Study the drawing (mm; zero at the part's minimum x, y, z) and answer. A direction names the side the tool comes from. Coordinates: 2 decimals unless noted, no trailing zeros. Loops run counter-clockwise (first coordinate to the right, second up) from the corner with the lowest first, then second, coordinate; pieces in that order, holes last.
Q1. Section C-C (x = 8.5) is taken. Give the vertices of the cut face in (y, z).
Q2. The mould has two halves that part along X. Classify the marked faces 3, 4 and 5: pulls with the +X half, pulls with the -X half, needs draft (parallel to the pull), parting line crosses it, or undercut.
Q3. Which of the six approach directions +Z, -Z, +X, -X, +Y, -Y give full straight-line access (tool end or side, diameter ignored) to the marked faces 1 and 2?
Q4. Flat-ended cylindrical pins translate along their axes: P1, Ø1.5, axis at x = 38, y = 18.5, coming from the +Z side; P2, Ø1.8, axis at x = 4, z = 21, coming from the +Y side; P3, Ø5, axis at x = 18.5, y = 4, coming from the +Z side; P4, Ø10.5, axis at x = 41.5, z = 14.5, coming from the +Y side. Find the tip coordinate at first contact, or state that the pin passes through.
Q5. Section A-A (y = 16) is taken. Give the vertices of the cut face in (x, z), then the cut area to 3 significant figures.
Q6. Section B-B (z = 23.5) is taken. Give the vertices of the cut face in (x, y).
Q7. Straight lines are drawn through the part: line 1 (X direction, y = 8.5, z = 28); line 2 (Y direction, x = 52, z = 4.5); line 3 (Y direction, x = 52, z = 20.5). For each, find the intervals that lie inside material, in ascending order.
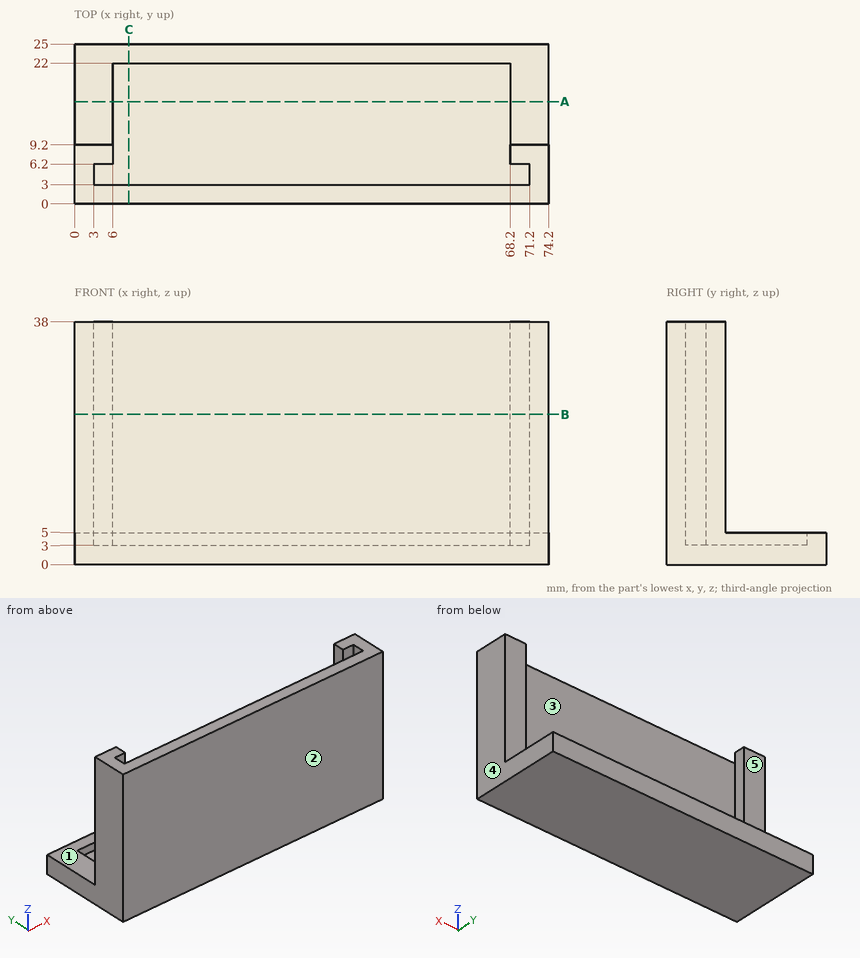
Numbers:
1. outline: (0, 0) - (25, 0) - (25, 5) - (22, 5) - (22, 3) - (3, 3) - (3, 38) - (0, 38) - close
2. face 3: undercut
2. face 4: pulls with the +X half
2. face 5: needs draft
3. face 1: +Z, +X, -X, +Y
3. face 2: +Z, -Z, +X, -X, -Y
4. P1: stops at z = 3
4. P2: stops at y = 9.2
4. P3: stops at z = 38
4. P4: stops at y = 3
5. outline: (0, 0) - (74.2, 0) - (74.2, 5) - (68.2, 5) - (68.2, 3) - (6, 3) - (6, 5) - (0, 5) - close
5. area: 247 mm2
6. outline: (0, 0) - (74.2, 0) - (74.2, 9.2) - (68.2, 9.2) - (68.2, 6.2) - (71.2, 6.2) - (71.2, 3) - (3, 3) - (3, 6.2) - (6, 6.2) - (6, 9.2) - (0, 9.2) - close
7. line 1: x = 0 to 6, 68.2 to 74.2
7. line 2: y = 0 to 3, 22 to 25
7. line 3: y = 0 to 3
